Read the model definition and answer for the solid it produces. Units are mm, in the model's axes. Face numbers are marked on the shaded views. A direction names the side the tool comes from. Coordinates: 2 decimals unless noted, no trailing zeros. Write each loop counter-clockwise with the first axis right and the second up, starting at its lowest first coordinate (ties: lowest second). Pieces come first, ordered by that corner, then holes. Notation, with made-up numbers: (16.5, 22.5) -> (20.5, 22.5) arc R35 ccw to (20.5, 61.5) -> close; hole circle Ø9 at (75, 45). An arc over 180 degrees is marked (long way). Answer as a JSON object with one key per item and string values. Group by question number.
(1) Which of the six approach directions +Z, -Z, +X, -X, +Y, -Y give full straight-line access (tool end or side, diameter ignored) to the marked faces 1, 2 and 3?
(2) Straight lines are drawn through the part: L1, parallel to Z at x = -2.5, y = 0.25; L2, parallel to X at y = -5, z = 2.25; L3, parallel to Z at x = 5.5, y = -2. For each, find the intervals that lie inside material, in ascending order.
(3) Find section D-D (y = 4.25). Give the vertices of the cut face in (x, z).
(4) Find section B-B (x = 1.75). Give the vertices of the cut face in (y, z), then the cut area to 3 significant figures.
(5) For a pull along Z with two mould halves and no side action, classify the marked faces 4, 5 and 6 as +Z half, -Z half, draft (parallel to the pull), parting line (faces both ways), or undercut.
(6) Find section A-A (y = -0.05). Give the vertices of the cut face in (x, z), then the cut area to 3 significant figures.
(7) Find section C-C (z = 2.5). Give the vertices of the cut face in (x, y), then the cut area to 3 significant figures.
from build123d import *

# Parameters (mm, degrees)
F0_W     = 15
F0_H     = 15
F1_DEPTH = 4
F2_W     = 10.5
F2_H     = 9.6
F2_R     = 1.25
F3_DEPTH = 2
F4_W     = 15
F4_H     = 15
F5_DEPTH = 3
F7_DEPTH = 15
F8_R     = 1
F9_SIZE  = 0.75


with BuildPart() as f1:
    # F0 (on Top) → F1 (new body)
    with BuildSketch(Plane.XY):
        Rectangle(F0_W, F0_H)
    extrude(amount=F1_DEPTH)

    # F2 (on face) → F3 (cut)
    with BuildSketch(Plane.XY.offset(4)):
        with Locations((0, -2.7)):
            Rectangle(F2_W, F2_H)
        with Locations((-2.7, -0.05)):
            Circle(F2_R, mode=Mode.SUBTRACT)
    extrude(amount=-F3_DEPTH, mode=Mode.SUBTRACT)

    # F4 (on face) → F5 (join)
    with BuildSketch(Plane(origin=(0, 0, 0), x_dir=(1, 0, 0), z_dir=(0, 0, -1))):
        Rectangle(F4_W, F4_H)
    extrude(amount=F5_DEPTH)

    # F6 (on face) → F7 (cut, through all)
    with BuildSketch(Plane.YZ.offset(7.5)):
        Polygon((-3.5, 0), (-6, -2), (6, -2), (3.5, 0), align=None)
    extrude(amount=-F7_DEPTH, mode=Mode.SUBTRACT)

    # F8
    f8_edges = [f1.edges().sort_by_distance(p)[0] for p in [
        (0, 7.5, 4),
        (-7.5, 0, 4),
        (7.5, 0, 4),
        (-6.375, -7.5, 4),
        (6.375, -7.5, 4),
        (-7.5, 7.5, 0.5),
        (-7.5, -7.5, 0.5),
        (7.5, -7.5, 0.5),
        (7.5, 7.5, 0.5),
    ]]
    fillet(f8_edges, radius=F8_R)

    # F9
    f9_edges = [f1.edges().sort_by_distance(p)[0] for p in [
        (5.25, -2.2, 4),
        (0, 2.1, 4),
        (-5.25, -2.2, 4),
    ]]
    chamfer(f9_edges, length=F9_SIZE)


solid = f1.part
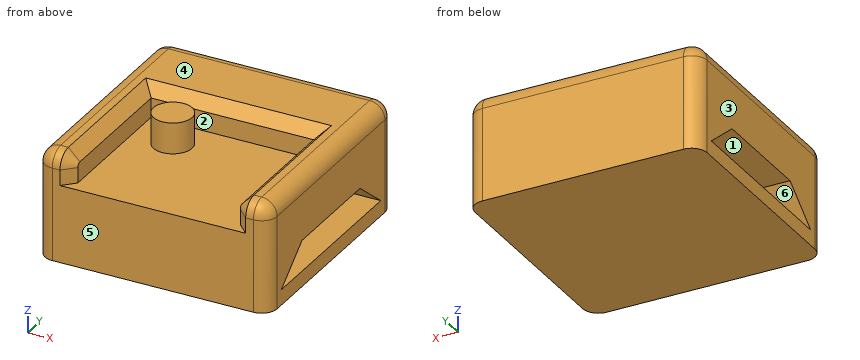
Results below:
{
 "1": {"face 1": "+X, -X", "face 2": "+Z", "face 3": "+Z, -Z, -X, +Y, -Y"},
 "2": {"L1": "z = -3 to -2, 0 to 4", "L2": "x = -7.5 to -5.25, 5.25 to 7.5", "L3": "z = -3 to -2, 0 to 3.5"},
 "3": {"outline": "(-7.5, -3) -> (7.5, -3) -> (7.5, -2) -> (-7.5, -2) -> close; (-7.5, -0.6) -> (7.5, -0.6) -> (7.5, 3) arc R1 ccw to (6.5, 4) -> (-6.5, 4) arc R1 ccw to (-7.5, 3) -> close"},
 "4": {"outline": "(-7.5, -3) -> (7.5, -3) -> (7.5, 3) arc R1 ccw to (6.5, 4) -> (2.85, 4) -> (2.1, 3.25) -> (2.1, 2) -> (-7.5, 2) -> close; hole (-6, -2) -> (6, -2) -> (3.5, 0) -> (-3.5, 0) -> close", "area": "66.3 mm2"},
 "5": {"face 4": "+Z half", "face 5": "draft", "face 6": "undercut"},
 "6": {"outline": "(-7.5, -3) -> (7.5, -3) -> (7.5, -2) -> (-7.5, -2) -> close; (-7.5, 0) -> (7.5, 0) -> (7.5, 3) arc R1 ccw to (6.5, 4) -> (6, 4) -> (5.25, 3.25) -> (5.25, 2) -> (-1.45, 2) -> (-1.45, 4) -> (-3.95, 4) -> (-3.95, 2) -> (-5.25, 2) -> (-5.25, 3.25) -> (-6, 4) -> (-6.5, 4) arc R1 ccw to (-7.5, 3) -> close", "area": "58.0 mm2"},
 "7": {"outline": "(-7.5, -6.5) arc R1 ccw to (-6.5, -7.5) -> (-6, -7.5) -> (-5.25, -6.75) -> (-5.25, 2.1) -> (5.25, 2.1) -> (5.25, -6.75) -> (6, -7.5) -> (6.5, -7.5) arc R1 ccw to (7.5, -6.5) -> (7.5, 6.5) arc R1 ccw to (6.5, 7.5) -> (-6.5, 7.5) arc R1 ccw to (-7.5, 6.5) -> close; circle Ø2.5 at (-2.7, -0.05)", "area": "128 mm2"}
}
